Here's how the part is built. I have some questions about the finished solid (model axes, mm). A direction names the side the tool comes from. Round coordinates to 2 decimals unless told otherwise and drop trailing zeros. Loops run counter-clockwise (first coordinate to the right, second up) from the corner with the lowest first, then second, coordinate; pieces in that order, holes last. Notation, with made-up numbers: (-27, 57) - (-9, 57) arc R21 ccw to (-9, 74) - close; hole circle Ø2 at (-30, 38.25). An arc over 180 degrees is marked (long way). Answer as a JSON object with one key per item and string values. Group by question number.
1) Which directions (+Z, -Z, +X, -X, +Y, -Y) give clear straight access to the entire face, cutting with the end or side of a thin tool? Please do faces 1 (the face through (0.6, 3, -1)), 2 (the face through (0.3, -2.71, 2.7)).
2) I want a section at A-A, the plane y = 0. Please give me the cut outline in (x, z) (3 decimals), then the cut area to 3 significant figures.
3) If we mould it in two halves opening along Y, with no side actions, what happens to faces 3 (the face through (0.3, -1.08, 4.88)), 4 (the face through (0.3, -2.7, -2.71)), 5 (the face through (0, 3, -1))? For each: pulls with the +Y half, pulls with the -Y half, needs draft (parallel to the pull), parting line crosses it, or undercut.
4) If I drill on line 1 along Z through (x, y) = (0.55, -2.75); line 2 along Y through (x, z) = (0.45, -1); line 3 along Z through (x, y) = (0.5, -0.25), over which ranges is the centre line in solid material (lowest first)? Write a range as [from, to].
Autodesk Inventor part; units mm, degrees
ref_plane "Work Plane1" through (0, 0, 0) normal (0, 1, 0) x (1, 0, 0)
ref_plane "YZ Plane" through (0, 0, 0) normal (1, 0, 0) x (0, 1, 0)
ref_plane "XZ Plane" through (0, 0, 0) normal (0, 1, 0) x (-1, 0, 0)
sketch "Sketch1" plane through (0, 0, 0) normal (1, 0, 0) x (0, 1, 0)
  circle A0 centre (0, 0) radius 5
  circle A1 centre (0, 0) radius 2.65
  dimension "d0" = 10
  dimension "d1" = 5.3
extrude "Body" add sketch "Sketch1" along normal blind 0.6
sketch "Sketch2" plane through (0, 0, 0) normal (-1, 0, 0) x (0, 0, 1)
  circle A0 centre (0, 0) radius 2.65
  circle A1 centre (0, 0) radius 5
  arc A2 (0.7462, 3.7515) -> (-0.7462, 3.7515) centre (0, 0) ccw
  line L0 (-0.517, 2.5991) -> (-0.7462, 3.7515)
  line L1 (0, 0) -> (0, 3.825) construction
  line L2 (0.517, 2.5991) -> (0.7462, 3.7515)
  line L3 (-0.517, 2.5991) -> (0, 0) construction
  line L4 (0.517, 2.5991) -> (0, 0) construction
  dimension "d4" = 7.65
  dimension "d5" = 11.25
extrude "Cut" cut sketch "Sketch2" against normal blind 0.6 contours A0 L0 A2 L2
fillet "Fillet1" radius 0.159 2 edges at (0.3, 3.7515, 0.7462) (0.3, 3.7515, -0.7462)
pattern_circular "Cuts" count 8 over 360 about axis through (-10, 0, 0) along (1, 0, 0) of "Cut", "Fillet1"
ref_plane "Work Plane1" through (0, 0, 0) normal (0, 1, 0) x (1, 0, 0)
equation "\"d0\" = SD2"
equation "\"d1\" = SD1"
equation "\"d2\" = SD"
equation "\"d4\" = 0.5 * SD2 + 0.5 * SD1"
equation "\"d6\" = SD"
equation "\"d8\" = 0.03 * SD1"
equation "\"SD1\" = 5.3"
equation "\"SD2\" = 10"
equation "\"SD\" = 0.6"
equation "\"NND\" = 5"
properties part number "DIN 6797 - J 5.3" material "Steel, Mild"
Outcome:
{
 "1": {"face 1": "+Z, -Z, +X, +Y, -Y", "face 2": "+X, -X"},
 "2": {"outline": "(0, -5) - (0.6, -5) - (0.6, -3.825) - (0, -3.825) - close; (0, 3.825) - (0.6, 3.825) - (0.6, 5) - (0, 5) - close", "area": "1.41 mm^2"},
 "3": {"face 3": "parting line crosses it", "face 4": "undercut", "face 5": "needs draft"},
 "4": {"line 1": "[-4.18, -2.66], [-1.84, -0.55], [0.55, 1.84], [2.66, 4.18]", "line 2": "[-4.9, -2.45], [2.45, 4.9]", "line 3": "[-4.99, -3.82], [3.82, 4.99]"}
}
